Read the model definition and answer for the solid it produces. Units are mm, in the model's axes. A direction names the side the tool comes from. Round coordinates to 2 decimals unless told otherwise and drop trailing zeros. Write each loop counter-clockwise with the first axis right and the second up, starting at its lowest first coordinate (ties: lowest second). Pieces come first, ordered by that corner, then holes. Notation, with made-up numbers: (75.5, -30) - (128.5, -30) arc R29 cw to (128.5, -8) - close; hole circle Ø6 at (-22, 76). An arc over 180 degrees is marked (long way). Answer as CSV lines item,"result". Start each with the question number.
1) Each of these flat-tipped pins is pushed along its axis until it touches: pin 1 (6 mm diameter, centred on x = 6.5, z = -3.5, fed in from -Y); pin 2 (1.5 mm diameter, centred on y = 1.5, z = -4, fed in from -X); pin 3 (1.5 mm diameter, centred on y = 1.5, z = -5, fed in from +X). Where does it stop, or does it pass through?
2) Find section B-B on x = 6. Determine the outline of the cut face in (y, z).
3) Consider line 1 along Y through (x, z) = (4.75, -4.5); line 2 along Y through (x, z) = (2, -5); line 3 along X through (y, z) = (1.5, -10.25). Determine where each line is inside the solid, lowest interval first.
4) Find section A-A on y = -1.75. Determine the outline of the cut face in (x, z), then the cut area to 3 significant figures.
5) For a pull along X with two mould halves and no side action, classify faces 1 (the flat face through (12.5, -1.5, -3.5)), 2 (the flat face through (6, 1, -12)), 3 (the flat face through (6, 0, -6)) as +X half, -X half, draft (parallel to the pull), parting line (faces both ways), or undercut.
6) Which of the six approach directions +Z, -Z, +X, -X, +Y, -Y give full straight-line access (tool end or side, diameter ignored) to faces 4 (the flat face through (0.5, 1.5, -11.5)), 5 (the flat face through (0, -1.7, -3.5)), 6 (the flat face through (1.5, 3.1, -6.1))?
7) Find section D-D on z = -6. Determine the outline of the cut face in (x, y).
8) Find section C-C on y = 2. Determine the outline of the cut face in (x, z), then the cut area to 3 significant figures.
from build123d import *

# Parameters (mm, degrees)
BOSS_EXTRU_2_DEPTH         = 3
ESQUISSE2_W                = 10
ESQUISSE2_H                = 10
BOSS_EXTRU_3_DEPTH         = 0.1
ESQUISSE3_R                = 4
BOSS_EXTRU_4_DEPTH         = 0.5
ESQUISSE4_W                = 1
ESQUISSE4_H                = 4
BOSS_EXTRU_5_DEPTH         = 0.5
ESQUISSE7_W                = 1
ESQUISSE7_H                = 4
BOSS_EXTRU_7_DEPTH         = 0.5
R_P_TITION_LIN_AIRE1_COUNT = 2
R_P_TITION_LIN_AIRE1_PITCH = 5


with BuildPart() as part:
    # Esquisse1 → Boss.-Extru.2 (new body)
    with BuildSketch(Plane(origin=(0, 0, 0), x_dir=(1, 0, 0), z_dir=(0, 1, 0))):
        Polygon((0, 11), (1, 12), (11, 12), (12, 11), (12, 1), (11, 0), (1, 0), (0, 1), align=None)
    extrude(amount=BOSS_EXTRU_2_DEPTH)

    # Esquisse2 → Boss.-Extru.3 (add)
    with BuildSketch(Plane(origin=(0, 3, 0), x_dir=(1, 0, 0), z_dir=(0, 1, 0))):
        with Locations((6, 6)):
            Rectangle(ESQUISSE2_W, ESQUISSE2_H)
    extrude(amount=BOSS_EXTRU_3_DEPTH)

    # Esquisse3 → Boss.-Extru.4 (add)
    with BuildSketch(Plane(origin=(0, 3.1, 0), x_dir=(1, 0, 0), z_dir=(0, 1, 0))):
        with Locations((6, 6)):
            Circle(ESQUISSE3_R)
    extrude(amount=BOSS_EXTRU_4_DEPTH)

    # Esquisse4 → Boss.-Extru.5 (add)
    with BuildSketch(Plane.ZY):
        with Locations((-8.5, -1.5)):
            Rectangle(ESQUISSE4_W, ESQUISSE4_H)
    boss_extru_5 = extrude(amount=BOSS_EXTRU_5_DEPTH)

    # Esquisse7 → Boss.-Extru.7 (add)
    with BuildSketch(Plane(origin=(12, 0, 0), x_dir=(0, 0, -1), z_dir=(1, 0, 0))):
        with Locations((8.5, -1.5)):
            Rectangle(ESQUISSE7_W, ESQUISSE7_H)
    boss_extru_7 = extrude(amount=BOSS_EXTRU_7_DEPTH)

    # Répétition linéaire1: Boss.-Extru.5, Boss.-Extru.7 ×2
    with Locations(*[(0, 0, i * R_P_TITION_LIN_AIRE1_PITCH) for i in range(1, R_P_TITION_LIN_AIRE1_COUNT)]):
        add(boss_extru_5)
        add(boss_extru_7)


solid = part.part
Check values:
1,pin 1,"stops at y = 0"
1,pin 2,"stops at x = 0"
1,pin 3,"stops at x = 12"
2,outline,"(0, -12) - (3, -12) - (3, -11) - (3.1, -11) - (3.1, -10) - (3.6, -10) - (3.6, -2) - (3.1, -2) - (3.1, -1) - (3, -1) - (3, 0) - (0, 0) - close"
3,line 1,"y = 0 to 3.6"
3,line 2,"y = 0 to 3.1"
3,line 3,"x = 0 to 12"
4,outline,"(-0.5, -9) - (0, -9) - (0, -8) - (-0.5, -8) - close; (-0.5, -4) - (0, -4) - (0, -3) - (-0.5, -3) - close; (12, -9) - (12.5, -9) - (12.5, -8) - (12, -8) - close; (12, -4) - (12.5, -4) - (12.5, -3) - (12, -3) - close"
4,area,"2.00 mm^2"
5,face 1,"+X half"
5,face 2,"draft"
5,face 3,"undercut"
6,face 4,"-Z, -X, +Y, -Y"
6,face 5,"+Z, -Z, -Y"
6,face 6,"+Y"
7,outline,"(0, 0) - (12, 0) - (12, 3) - (11, 3) - (11, 3.1) - (10, 3.1) - (10, 3.6) - (2, 3.6) - (2, 3.1) - (1, 3.1) - (1, 3) - (0, 3) - close"
8,outline,"(0, -11) - (1, -12) - (11, -12) - (12, -11) - (12, -1) - (11, 0) - (1, 0) - (0, -1) - close"
8,area,"142 mm^2"
